from build123d import *

# Parameters (mm, degrees)
ESQUISSE1_R             = 1.7
ESQUISSE1_R_2           = 3
ESQUISSE1_R_3           = 1.4
BOSS_EXTRU_1_DEPTH      = 3
ESQUISSE1_3_R           = 2.4
ESQUISSE1_3_R_2         = 1.4
ENL_V_MAT_EXTRU_1_DEPTH = 2


with BuildPart() as part:
    # Esquisse1 → Boss.-Extru.1 (new body)
    with BuildSketch(Plane(origin=(0, 0, 0), x_dir=(1, 0, 0), z_dir=(0, 1, 0))):
        Polygon((19.5, 48), (-45.5, 48), (-45.5, 18.5), (-22, 18.5), (-22, -9.5), (-45.5, -9.5), (-45.5, -48), (19.5, -48), align=None)
        with Locations(Location((16.5, -43.5, 0), (0, 0, 270))):
            Circle(ESQUISSE1_R, mode=Mode.SUBTRACT)
        with Locations(Location((7.5, 44.5, 0), (0, 0, 270))):
            Circle(ESQUISSE1_R, mode=Mode.SUBTRACT)
        with Locations(Location((-7.5, 44.5, 0), (0, 0, 270))):
            Circle(ESQUISSE1_R, mode=Mode.SUBTRACT)
        with Locations(Location((-13.5, -43.5, 0), (0, 0, 270))):
            Circle(ESQUISSE1_R_2, mode=Mode.SUBTRACT)
        with Locations(Location((-41.5, -20.5, 0), (0, 0, 270))):
            Circle(ESQUISSE1_R_3, mode=Mode.SUBTRACT)
        with Locations(Location((7.5, -20.5, 0), (0, 0, 270))):
            Circle(ESQUISSE1_R_3, mode=Mode.SUBTRACT)
        with Locations(Location((7.5, 37.5, 0), (0, 0, 270))):
            Circle(ESQUISSE1_R_3, mode=Mode.SUBTRACT)
        with Locations(Location((-41.5, 37.5, 0), (0, 0, 270))):
            Circle(ESQUISSE1_R_3, mode=Mode.SUBTRACT)
    extrude(amount=BOSS_EXTRU_1_DEPTH)

    # Esquisse1<3> → Enlèv. mat.-Extru.1 (cut)
    # profile 1 of 4: a face of its own
    with BuildSketch(Plane(origin=(0, 0, 0), x_dir=(1, 0, 0), z_dir=(0, 1, 0))):
        with Locations(Location((-41.5, -20.5, 0), (0, 0, 270))):
            Circle(ESQUISSE1_3_R)
        with Locations(Location((-41.5, -20.5, 0), (0, 0, 270))):
            Circle(ESQUISSE1_3_R_2, mode=Mode.SUBTRACT)
    # profile 2 of 4: a face of its own
    with BuildSketch(Plane(origin=(0, 0, 0), x_dir=(1, 0, 0), z_dir=(0, 1, 0))):
        with Locations(Location((7.5, -20.5, 0), (0, 0, 270))):
            Circle(ESQUISSE1_3_R)
        with Locations(Location((7.5, -20.5, 0), (0, 0, 270))):
            Circle(ESQUISSE1_3_R_2, mode=Mode.SUBTRACT)
    # profile 3 of 4: a face of its own
    with BuildSketch(Plane(origin=(0, 0, 0), x_dir=(1, 0, 0), z_dir=(0, 1, 0))):
        with Locations(Location((7.5, 37.5, 0), (0, 0, 270))):
            Circle(ESQUISSE1_3_R)
        with Locations(Location((7.5, 37.5, 0), (0, 0, 270))):
            Circle(ESQUISSE1_3_R_2, mode=Mode.SUBTRACT)
    # profile 4 of 4: a face of its own
    with BuildSketch(Plane(origin=(0, 0, 0), x_dir=(1, 0, 0), z_dir=(0, 1, 0))):
        with Locations(Location((-41.5, 37.5, 0), (0, 0, 270))):
            Circle(ESQUISSE1_3_R)
        with Locations(Location((-41.5, 37.5, 0), (0, 0, 270))):
            Circle(ESQUISSE1_3_R_2, mode=Mode.SUBTRACT)
    extrude(amount=ENL_V_MAT_EXTRU_1_DEPTH, mode=Mode.SUBTRACT)


solid = part.part
Model file for the job. Use its own axes, mm. A direction names the side the tool comes from. Give positions to 0.01 mm unless a question says otherwise; leave off trailing zeros. Loops run counter-clockwise (first coordinate to the right, second up) from the corner with the lowest first, then second, coordinate; pieces in that order, holes last.
1) Pull direction Z, two halves, no side cores. Call faces 4 (the flat face through (-34, 1, -18.5)), 5 (the flat face through (-43, 2, -36)), 6 (the flat face through (-13, 1, 48)), 7 (the flat face through (-45.5, 1, 28)): +Z half, -Z half, draft (parallel to the pull), parting line (faces both ways), or undercut.
2) Saw through at C-C (y = 1.3). Count the separate pieces of the cut face and the enclosed holes in it, plus the area to 3 significant figures.
3) Saw through at A-A (x = 7.5). Write the cut outline in (y, z).
4) Saw through at D-D (x = -13.5). Write the cut outline in (y, z), plus the area to 3 significant figures.
5) Wall check: line 1 (X direction, y = 2.3, z = 20.5); line 2 (X direction, y = 1.8, z = 43.5); line 3 (Z direction, x = -30, y = 0.6). Give the ranges that are in metal, low to high.
6) Saw through at B-B (z = -44.5). Write the cut outline in (x, y), plus the area to 3 significant figures.
7) Flat gauge pins, fed straight in: pin 1 Ø3.5 at (x, z) = (-41.5, 20.5) entering from -Y; pin 2 Ø1.5 at (y, z) = (1, -2.5) entering from -X. Where does each tip first touch, or does it go through?
8) Tool access for faces 1 (the flat face through (-34, 1, 9.5)), 2 (the cylindrical face through (-40.11, 2.49, -37.68)), 3 (the cylindrical face through (-43.843, 0.986, -38.02)): list every direction of +Z, -Z, +X, -X, +Y, -Y with a clear straight run to the whole face (end or side of a thin tool).
Answer block:
1. face 4: undercut
1. face 5: undercut
1. face 6: +Z half
1. face 7: draft
2. separate pieces: 1
2. enclosed holes: 8
2. area: 5,450 mm2
3. outline: (0, -48) - (3, -48) - (3, -46.2) - (0, -46.2) - close; (0, -42.8) - (3, -42.8) - (3, -38.9) - (2, -38.9) - (2, -39.9) - (0, -39.9) - close; (0, -35.1) - (2, -35.1) - (2, -36.1) - (3, -36.1) - (3, 19.1) - (2, 19.1) - (2, 18.1) - (0, 18.1) - close; (0, 22.9) - (2, 22.9) - (2, 21.9) - (3, 21.9) - (3, 48) - (0, 48) - close
4. outline: (0, -48) - (3, -48) - (3, 40.5) - (0, 40.5) - close; (0, 46.5) - (3, 46.5) - (3, 48) - (0, 48) - close
4. area: 270 mm2
5. line 1: x = -45.5 to -42.9, -40.1 to 6.1, 8.9 to 19.5
5. line 2: x = -45.5 to -16.5, -10.5 to 14.8, 18.2 to 19.5
5. line 3: z = -48 to -18.5, 9.5 to 48
6. outline: (-45.5, 0) - (-9.2, 0) - (-9.2, 3) - (-45.5, 3) - close; (-5.8, 0) - (5.8, 0) - (5.8, 3) - (-5.8, 3) - close; (9.2, 0) - (19.5, 0) - (19.5, 3) - (9.2, 3) - close
6. area: 175 mm2
7. pin 1: stops at y = 2
7. pin 2: stops at x = -22
8. face 1: -X, +Y, -Y
8. face 2: +Y, -Y
8. face 3: -Y
